Can you work these out from the model? Positions are in its coordinate system, mm. Give positions to 0.01 mm unless a question says otherwise; leave off trailing zeros. Order: outer loops, then holes, each group sorted by start corner. A loop starts at its lowest first (then second) coordinate and runs counter-clockwise, first axis right, second up. Notation, with made-up numbers: M 55.25,-23.75 L 81.25,-23.75 A8 ccw 81.25,-15.75 Z; hole C 45.25,62.5 d6. An arc over 180 degrees is marked long. Answer as a JSON object with one key per item and string values.
```python
from build123d import *

# Parameters (mm, degrees)
F1_DEPTH       = 5.08
F3_D           = 6.35
F3_CSINK_D     = 12.7
F3_CSINK_ANGLE = 90


with BuildPart() as f1:
    # F0 (on Top) → F1 (new body)
    with BuildSketch(Plane.XY):
        with BuildLine():
            ThreePointArc((2.0111581622, -26.8418043852), (19.731467902, -18.3083695134), (26.9170432961, 0))
            ThreePointArc((26.9170432961, 0), (19.0332238442, 19.0332238442), (0, 26.9170432961))
            Line((0, 26.9170432961), (0, -26.8418043852))
            Line((0, -26.8418043852), (2.0111581622, -26.8418043852))
        make_face()
        with BuildLine():
            ThreePointArc((0, 26.9170432961), (19.0332238442, 19.0332238442), (26.9170432961, 0))
            ThreePointArc((26.9170432961, 0), (19.731467902, -18.3083695134), (2.0111581622, -26.8418043852))
            Line((2.0111581622, -26.8418043852), (69.3475157022, -26.8418043852))
            Line((69.3475157022, -26.8418043852), (69.3475157022, 26.9170432961))
            Line((69.3475157022, 26.9170432961), (0, 26.9170432961))
        make_face()
        with BuildLine():
            Line((0, -26.8418043852), (0, 26.9170432961))
            ThreePointArc((0, 26.9170432961), (-26.8982269916, -1.0062825209), (2.0111581622, -26.8418043852))
            Line((2.0111581622, -26.8418043852), (0, -26.8418043852))
        make_face()
    extrude(amount=F1_DEPTH)

    # F3 (through all)
    with Locations(Plane.XY.offset(5.08)):
        with Locations((0, 0)):
            CounterSinkHole(F3_D / 2, F3_CSINK_D / 2, counter_sink_angle=F3_CSINK_ANGLE)


solid = f1.part
```
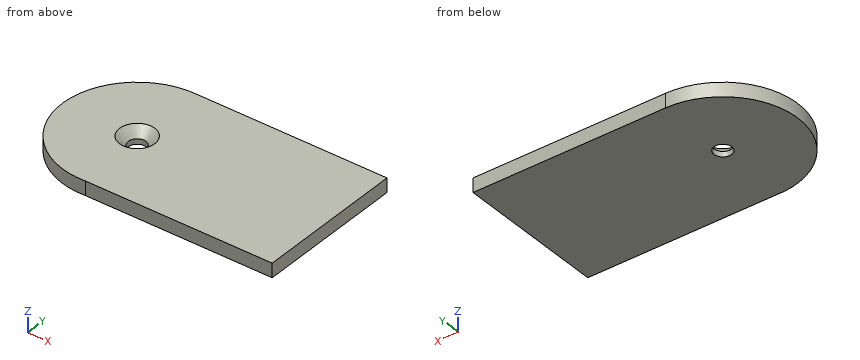
1) I need wall thicknesses on L1, parallel to X at y = 0, z = 0.4 (3 decimals); L2, parallel to Y at x = 0, z = 0.8 (3 decimals); L3, parallel to Y at x = 21.5, z = 0.95. Which ranges of each line are inside material? Lowest first, please.
Results found:
{"L1": "x = -26.917 to -3.175, 3.175 to 69.348", "L2": "y = -26.917 to -3.175, 3.175 to 26.917", "L3": "y = -26.84 to 26.92"}
2) I want a section at B-B on y = -20.5. Write out the boundary of the cut face in (x, z).
Results found:
{"outline": "M -17.44,0 L 69.35,0 L 69.35,5.08 L -17.44,5.08 Z"}
3) I want a section at A-A on y = 0. Write out the boundary of the cut face in (x, z) (3 decimals), and give its area (3 significant figures).
Results found:
{"outline": "M -26.917,0 L -3.175,0 L -3.175,1.905 L -6.35,5.08 L -26.917,5.08 Z; M 3.175,0 L 69.348,0 L 69.348,5.08 L 6.35,5.08 L 3.175,1.905 Z", "area": "447 mm²"}
4) I'm going to push flat-ended pins straight in: pin 1 Ø2 at (y, z) = (7, 2.5) entering from -X; pin 2 Ø2.5 at (x, z) = (30.5, 1.5) entering from -Y. Where does each tip first touch, or does it pass through?
Results found:
{"pin 1": "stops at x = -26.24", "pin 2": "stops at y = -26.84"}
5) I want a section at C-C on y = -9. Write out the boundary of the cut face in (x, z).
Results found:
{"outline": "M -25.37,0 L 69.35,0 L 69.35,5.08 L -25.37,5.08 Z"}
